For this review, take the finished solid that the model builds, in its own axes (mm). Round coordinates to 2 decimals unless told otherwise and drop trailing zeros. Write each loop counter-clockwise with the first axis right and the second up, starting at its lowest first coordinate (ties: lowest second). Pieces come first, ordered by that corner, then holes. Notation, with made-up numbers: M -7.5,-17.75 L 20.5,-17.75 A30 ccw 20.5,14.25 Z; hole C 6.25,33.5 d11. An arc over 180 degrees is marked long. Answer in a Markdown table with one row per item.
```python
from build123d import *

# Parameters (mm, degrees)
ESQUISSE1_W             = 149
ESQUISSE1_H             = 10
BOSS_EXTRU_1_DEPTH      = 3
ESQUISSE2_R             = 1.005
ESQUISSE2_W             = 5
ESQUISSE2_H             = 3
ENL_V_MAT_EXTRU_1_DEPTH = 150.365323954


with BuildPart() as part:
    # Esquisse1 → Boss.-Extru.1 (new body)
    with BuildSketch(Plane.XY):
        with Locations((74.5, 5)):
            Rectangle(ESQUISSE1_W, ESQUISSE1_H)
    extrude(amount=BOSS_EXTRU_1_DEPTH)

    # Esquisse2 → Enlèv. mat.-Extru.1 (cut, through all)
    with BuildSketch(Plane(origin=(0, 0, 0), x_dir=(-1, 0, 0), z_dir=(0, 0, -1))):
        with Locations((-3, 3)):
            Circle(ESQUISSE2_R)
        with Locations((-146, 3)):
            Circle(ESQUISSE2_R)
        with Locations((-141.5, 6.5)):
            Rectangle(ESQUISSE2_W, ESQUISSE2_H)
        with Locations((-131.5, 6.5)):
            Rectangle(ESQUISSE2_W, ESQUISSE2_H)
        with Locations((-121.5, 6.5)):
            Rectangle(ESQUISSE2_W, ESQUISSE2_H)
        with Locations((-111.5, 6.5)):
            Rectangle(ESQUISSE2_W, ESQUISSE2_H)
        with Locations((-101.5, 6.5)):
            Rectangle(ESQUISSE2_W, ESQUISSE2_H)
        with Locations((-91.5, 6.5)):
            Rectangle(ESQUISSE2_W, ESQUISSE2_H)
        with Locations((-81.5, 6.5)):
            Rectangle(ESQUISSE2_W, ESQUISSE2_H)
        with Locations((-71.5, 6.5)):
            Rectangle(ESQUISSE2_W, ESQUISSE2_H)
        with Locations((-61.5, 6.5)):
            Rectangle(ESQUISSE2_W, ESQUISSE2_H)
        with Locations((-51.5, 6.5)):
            Rectangle(ESQUISSE2_W, ESQUISSE2_H)
        with Locations((-41.5, 6.5)):
            Rectangle(ESQUISSE2_W, ESQUISSE2_H)
        with Locations((-31.5, 6.5)):
            Rectangle(ESQUISSE2_W, ESQUISSE2_H)
        with Locations((-21.5, 6.5)):
            Rectangle(ESQUISSE2_W, ESQUISSE2_H)
        with Locations((-11.5, 6.5)):
            Rectangle(ESQUISSE2_W, ESQUISSE2_H)
    extrude(amount=-ENL_V_MAT_EXTRU_1_DEPTH, mode=Mode.SUBTRACT)


solid = part.part
```
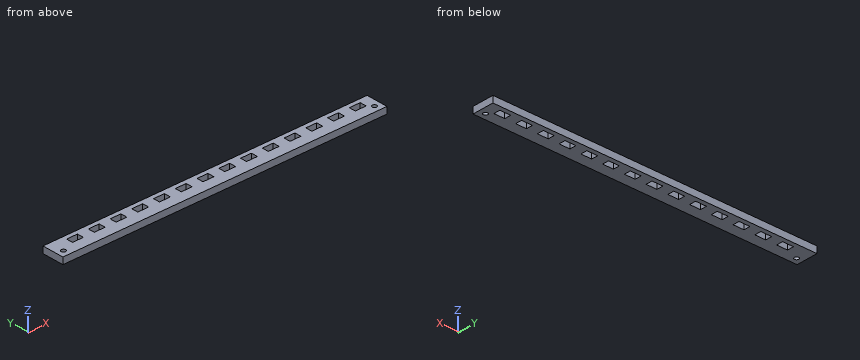
Q1. Take a section at A-A (x = 92). State the section outline as (y, z) points, then the cut area to 3 significant figures.
Found:
| item | result |
|---|---|
| outline | M 0,0 L 5,0 L 5,3 L 0,3 Z; M 8,0 L 10,0 L 10,3 L 8,3 Z |
| area | 21.0 mm² |
Q2. Take a section at B-B (z = 2.3). State how many separate pieces and enclosed holes the cut face has, then the cut area to 3 significant figures.
Found:
| item | result |
|---|---|
| separate pieces | 1 |
| enclosed holes | 16 |
| area | 1,270 mm² |
Q3. For probe 1 along Y at (x, z) = (3, 1.75) (3 decimals); probe 2 along Y at (x, z) = (21, 0.15), list the stretches that pass through material, from the lowest coordinate up.
Found:
| item | result |
|---|---|
| probe 1 | 0 to 1.995, 4.005 to 10 |
| probe 2 | 0 to 5, 8 to 10 |
